Part model, mm, in its own coordinate system. A direction names the side the tool comes from. Give positions to 0.01 mm unless a question says otherwise; leave off trailing zeros. Write each loop counter-clockwise with the first axis right and the second up, starting at its lowest first coordinate (ties: lowest second). Pieces come first, ordered by that corner, then holes.
Autodesk Inventor part; units mm, degrees
ref_plane "YZ Plane" through (0, 0, 0) normal (1, 0, 0) x (0, 1, 0)
ref_plane "XZ Plane" through (0, 0, 0) normal (0, 1, 0) x (-1, 0, 0)
ref_plane "XY Plane" through (0, 0, 0) normal (0, 0, 1) x (1, 0, 0)
sketch "Эскиз1" plane through (0, 0, 0) normal (0, 0, 1) x (1, 0, 0)
  line L0 (69.1759, 4.9444) -> (70.4259, 4.9444)
  line L1 (70.4259, 4.9444) -> (70.4259, 2.9444)
  line L2 (67.4259, 4.9444) -> (67.4259, 0)
  line L3 (69.1759, 4.9444) -> (69.1759, 1.9444)
  line L4 (70.4259, 2.9444) -> (71.4259, 2.9444)
  line L5 (71.4259, 2.9444) -> (71.4259, -1.0556)
  line L6 (71.4259, -1.0556) -> (70.6259, -1.0556)
  line L7 (70.6259, -1.0556) -> (69.1759, 1.9444)
  point P0 (0, 0)
  dimension "d0" = 6
  dimension "d1" = 8
  dimension "d2" = 2
  dimension "d3" = 4
  dimension "d4" = 3
  dimension "d5" = 0.8
  dimension "d6" = 3.5
revolve "Вращение1" add sketch "Эскиз1" angle 360 about axis through (67.4259, 4.9444, 0) along (0, -1, 0)
chamfer "Фаска1" distance 0.5 angle 45 1 edges at (65.6759, 4.9444, 0)
properties part number "nut" material "Сталь, литейная"
1) 3-axis set-ups, long thin cutter, end or side, ignore diameter. For faces 1 (the cylindrical face through (70.287, 3.93, 0.901)), 2 (the flat face through (69, -1.056, 3)): which of +Z, -Z, +X, -X, +Y, -Y reach the whole face in a straight line?
Check result:
face 1: +Y
face 2: +Z, -Z, +X, -X, -Y
2) Saw through at A-A (z = 0). Write the cut outline in (x, y), and give its area (3 significant figures).
Check result:
outline: (63.43, -1.06) - (64.23, -1.06) - (65.68, 1.94) - (65.68, 4.44) - (65.18, 4.94) - (64.43, 4.94) - (64.43, 2.94) - (63.43, 2.94) - close; (69.18, 1.94) - (70.63, -1.06) - (71.43, -1.06) - (71.43, 2.94) - (70.43, 2.94) - (70.43, 4.94) - (69.68, 4.94) - (69.18, 4.44) - close
area: 18.4 mm2
3) Drill centre lines: L1, parallel to Y at x = 64, z = -2; L2, parallel to Z at x = 69, y = -0.15; L3, parallel to Z at x = 68.25, y = -0.4. Where is each one in solid material? Low to high.
Check result:
L1: y = -1.06 to 2.94
L2: z = -3.68 to -2.27, 2.27 to 3.68
L3: z = -3.91 to -2.76, 2.76 to 3.91
4) Flat gauge pins, fed straight in: P1, Ø1, axis at y = 3.5, z = -2.5, coming from the +X side; P2, Ø3, axis at x = 67.43, z = 0, coming from the +Y side. Where does each tip first touch, or does it go through?
Check result:
P1: stops at x = 69.66
P2: passes through
5) Saw through at B-B (y = 3.7). Write the cut outline in (x, z), and give its area (3 significant figures).
Check result:
outline: circle Ø6 at (67.43, 0); hole circle Ø3.5 at (67.43, 0)
area: 18.7 mm2
6) Mould opens along Z. For faces 3 (the cylindrical face through (69.095, 3.177, 0.526)), 4 (the flat face through (69, 4.944, 2)), 5 (the cylindrical face through (63.43, 0.92, 0.18)) say: +Z half, -Z half, draft (parallel to the pull), parting line (faces both ways), or undercut.
Check result:
face 3: undercut
face 4: draft
face 5: parting line
7) Saw through at C-C (y = 2.3). Write the cut outline in (x, z), and give its area (3 significant figures).
Check result:
outline: circle Ø8 at (67.43, 0); hole circle Ø3.5 at (67.43, 0)
area: 40.6 mm2
